The drawing under review shows one solid part. Ordinate dimensions are in mm from its lowest x, y, z. A direction names the side the tool comes from. Give positions to 0.01 mm unless a question says otherwise; leave off trailing zeros. Order: outer loops, then holes, each group sorted by start corner. A loop starts at its lowest first (then second) coordinate and runs counter-clockwise, first axis right, second up. Notation, with made-up numbers: (75, -19.5) - (85, -19.5) arc R7 cw to (85, -12.5) - close; hole circle Ø8 at (3, -7). An arc over 180 degrees is marked (long way). Answer as a JSON object with one key per item and string values. Group by question number.
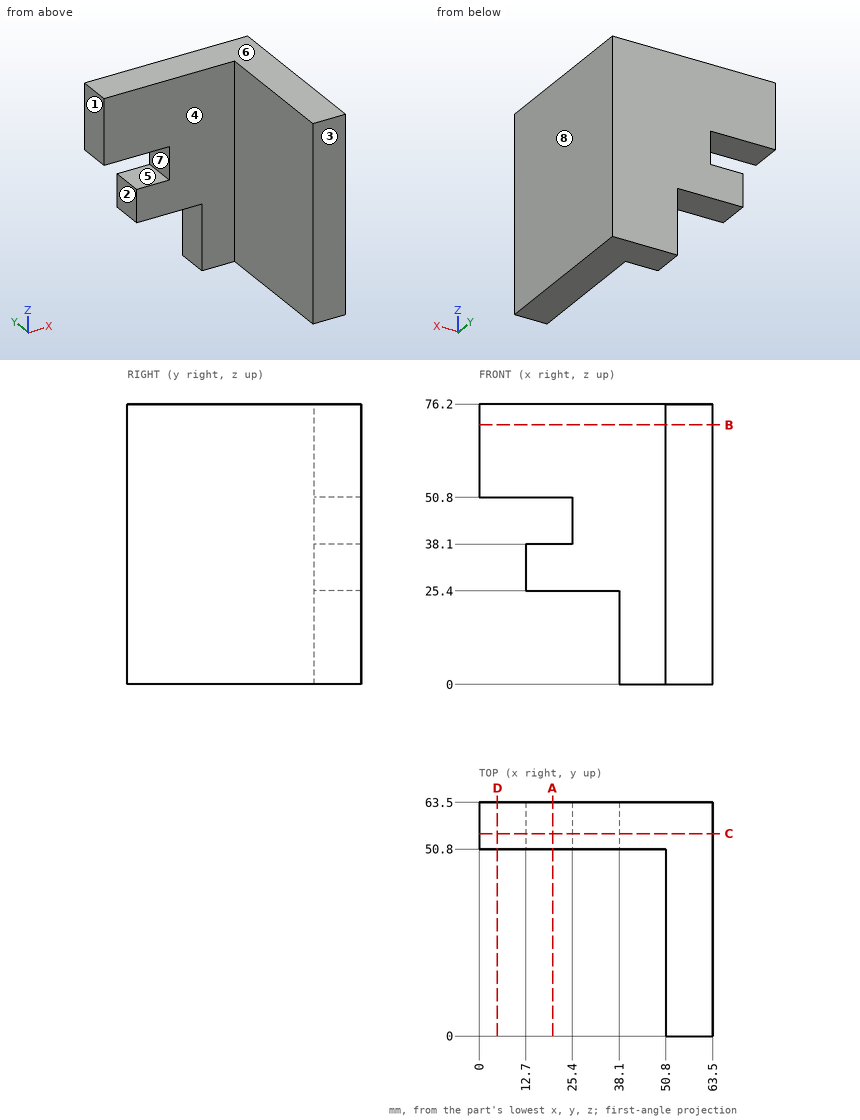
1) Consider section A-A (x = 20). Give the boundary of the cut face in (y, z), plus the area to 3 significant figures.
2) For the marked faces 1, 2, 3, 4 and 5, list the 3-axis set-ups (+Z, -Z, +X, -X, +Y, -Y) from which the entire face can be reached by the end or side of a thin tool; tool diameter is ignored.
3) Consider section B-B (z = 70.5). Give the boundary of the cut face in (x, y).
4) For line 1 (Z direction, x = 14.5, y = 53); line 2 (X direction, y = 57, z = 40.5); line 3 (X direction, y = 4, z = 31.5), list the stretches that pass through material, from the lowest coordinate up.
5) Consider section D-D (x = 5). Give the boundary of the cut face in (y, z), plus the area to 3 significant figures.
6) Consider section C-C (y = 55). Give the boundary of the cut face in (x, z).
7) For pin 1 (10 mm diameter, centred on y = 58, z = 17, fed in from -X); pin 2 (4 mm diameter, centred on x = 7.5, y = 54.5, fed in from -Z); pin 3 (4 mm diameter, centred on y = 60.5, z = 47, fed in from -X), all flat-tipped, find the tip position at first contact; note any pin that passes through.
8) Mouldability with a two-part tool opening along Z and no side actions: class the marked faces 6, 7 and 8 as released by +Z, released by -Z, zero draft, split by the parting line, or undercut.
Result set:
{
 "1": {"outline": "(50.8, 25.4) - (63.5, 25.4) - (63.5, 38.1) - (50.8, 38.1) - close; (50.8, 50.8) - (63.5, 50.8) - (63.5, 76.2) - (50.8, 76.2) - close", "area": "484 mm2"},
 "2": {"face 1": "+Z, -Z, -X, +Y, -Y", "face 2": "-Z, -X, +Y, -Y", "face 3": "+Z, -Z, +X, -X, -Y", "face 4": "+Z, -Z, -X, -Y", "face 5": "-X, +Y, -Y"},
 "3": {"outline": "(0, 50.8) - (50.8, 50.8) - (50.8, 0) - (63.5, 0) - (63.5, 63.5) - (0, 63.5) - close"},
 "4": {"line 1": "z = 25.4 to 38.1, 50.8 to 76.2", "line 2": "x = 25.4 to 63.5", "line 3": "x = 50.8 to 63.5"},
 "5": {"outline": "(50.8, 50.8) - (63.5, 50.8) - (63.5, 76.2) - (50.8, 76.2) - close", "area": "323 mm2"},
 "6": {"outline": "(0, 50.8) - (25.4, 50.8) - (25.4, 38.1) - (12.7, 38.1) - (12.7, 25.4) - (38.1, 25.4) - (38.1, 0) - (63.5, 0) - (63.5, 76.2) - (0, 76.2) - close"},
 "7": {"pin 1": "stops at x = 38.1", "pin 2": "stops at z = 50.8", "pin 3": "stops at x = 25.4"},
 "8": {"face 6": "released by +Z", "face 7": "undercut", "face 8": "zero draft"}
}
